Work out the finished part from the listing and answer in its coordinate system (mm). A direction names the side the tool comes from. Coordinates: 2 decimals unless noted, no trailing zeros. Write each loop counter-clockwise with the first axis right and the second up, starting at its lowest first coordinate (ties: lowest second). Pieces come first, ordered by that corner, then holes. Notation, with made-up numbers: (64.5, 23) - (92.5, 23) arc R14 ccw to (92.5, 48) - close; hole circle Ø3 at (7.5, 76.5). An arc over 180 degrees is marked (long way). Answer as a JSON object with one key per item and string values. Group by question number.
from build123d import *

# Parameters (mm, degrees)
SKETCH1_R           = 1.5999999999999992
SKETCH1_R_2         = 1.6
BOSS_EXTRUDE1_DEPTH = 1.5
BOSS_EXTRUDE2_DEPTH = 20
FILLET1_R           = 5
SKETCH2_R           = 1.6500000000000017
SKETCH2_W           = 42.900000000000006
SKETCH2_H           = 21.999999999999993
CUT_EXTRUDE1_DEPTH  = 191.86971996626394
FILLET2_R           = 2


with BuildPart() as part:
    # Sketch1 → Boss-Extrude1 (new, symmetric)
    with BuildSketch(Plane(origin=(0, 0, 0), x_dir=(1, 0, 0), z_dir=(0, 1, 0))):
        Polygon((-15, -39), (-15, 39), (-14.999999999999993, 64), (5.358274547724965, 122.5), (119.64234676884817, 122.50000000000003), (145.00000000000003, 86.28551808227317), (145.00000000000003, -86.28551808227317), (119.64234676884817, -122.50000000000003), (5.358274547725049, -122.49999999999999), (-14.999999999999993, -64), align=None)
        with Locations(Location((0, 31, 0), (0, 0, 270))):
            Circle(SKETCH1_R, mode=Mode.SUBTRACT)
        with Locations(Location((0, -31, 0), (0, 0, 90))):
            Circle(SKETCH1_R_2, mode=Mode.SUBTRACT)
        Polygon((25.197972880423116, 27.499999999999996), (128, 27.499999999999996), (128, 80.92543867133034), (110.7927069094685, 105.50000000000004), (17.442194764625423, 105.50000000000001), (3.0000000000000027, 64), (3.0000000000000027, 39), align=None, mode=Mode.SUBTRACT)
        Polygon((25.197972880423116, -27.499999999999996), (128, -27.499999999999996), (128, -80.92543867133034), (110.7927069094685, -105.50000000000004), (17.442194764625537, -105.49999999999999), (3.0000000000000027, -64), (3.0000000000000027, -39), align=None, mode=Mode.SUBTRACT)
    extrude(amount=BOSS_EXTRUDE1_DEPTH, both=True)

    # Sketch3 → Boss-Extrude2 (add)
    with BuildSketch(Plane(origin=(0, 1.5, 0), x_dir=(1, 0, 0), z_dir=(0, 1, 0))):
        Polygon((120.00000000000004, -2.999999999999993), (120.00000000000004, 3.0000000000000075), (138, 3.0000000000000075), (138, 84.07842656012029), (115.99837741498601, 115.49999999999999), (10.334006401742785, 115.49999999999997), (-4.464169294218266, 72.97708008435012), (-11.07528040532939, 75.27777777777771), (5.358274547724965, 122.5), (119.64234676884817, 122.50000000000003), (145.00000000000003, 86.28551808227317), (145.00000000000003, -86.28551808227317), (119.64234676884817, -122.50000000000003), (5.358274547724965, -122.5), (-11.075280405329384, -75.27777777777771), (-4.464169294218257, -72.97708008435012), (10.334006401742798, -115.49999999999997), (115.99837741498602, -115.49999999999996), (138, -84.07842656012026), (138, -2.999999999999991), align=None)
    extrude(amount=BOSS_EXTRUDE2_DEPTH)

    # Fillet1
    fillet1_edges = [part.edges().sort_by_distance(p)[0] for p in [
        (115.99837741498602, 11.5, 115.49999999999996),
        (10.334006401742798, 11.5, 115.49999999999997),
        (-11.075280405329384, 11.5, 75.27777777777771),
        (-11.07528040532939, 11.5, -75.27777777777771),
        (10.334006401742785, 11.5, -115.49999999999997),
        (115.99837741498601, 11.5, -115.49999999999999),
        (138, 11.5, -84.07842656012029),
        (5.358274547724965, 10, -122.5),
        (119.64234676884817, 10, -122.50000000000003),
        (145.00000000000003, 10, -86.28551808227317),
        (145.00000000000003, 10, 86.28551808227317),
        (119.64234676884817, 10, 122.50000000000003),
        (5.358274547725006, 10, 122.5),
        (128, 0, -80.92543867133034),
        (110.7927069094685, 0, -105.50000000000004),
        (17.442194764625423, 0, -105.50000000000001),
        (138, 11.5, -3.0000000000000075),
        (138, 11.5, 2.999999999999991),
        (138, 11.5, 84.07842656012026),
    ]]
    fillet(fillet1_edges, radius=FILLET1_R)

    # Sketch2 → Cut-Extrude1 (cut, through all)
    with BuildSketch(Plane(origin=(0, 1.5, 0), x_dir=(1, 0, 0), z_dir=(0, 1, 0))):
        with Locations(Location((56.999999999999964, 18.99999999999999, 0), (0, 0, 270))):
            Circle(SKETCH2_R)
        with Locations(Location((84.99999999999997, 18.999999999999993, 0), (0, 0, 270))):
            Circle(SKETCH2_R)
        with Locations(Location((101.99999999999999, 16.999999999999996, 0), (0, 0, 270))):
            Circle(SKETCH2_R)
        with Locations(Location((101.99999999999999, -16.999999999999996, 0), (0, 0, 90))):
            Circle(SKETCH2_R)
        with Locations(Location((84.99999999999997, -18.999999999999993, 0), (0, 0, 90))):
            Circle(SKETCH2_R)
        with Locations(Location((56.999999999999964, -18.99999999999999, 0), (0, 0, 90))):
            Circle(SKETCH2_R)
        with Locations((81.24999999999999, 3.819e-14)):
            Rectangle(SKETCH2_W, SKETCH2_H)
    extrude(amount=-CUT_EXTRUDE1_DEPTH, mode=Mode.SUBTRACT)

    # Fillet2
    fillet2_edges = [part.edges().sort_by_distance(p)[0] for p in [
        (59.79999999999998, 0, -11.000000000000036),
        (102.69999999999999, 0, -11.000000000000036),
        (102.69999999999999, 0, 10.99999999999996),
        (59.79999999999998, 0, 10.99999999999996),
    ]]
    fillet(fillet2_edges, radius=FILLET2_R)


solid = part.part
Q1. Section C-C on z = -36 is taken. Determine the outline of the cut face in (x, y), plus the area to 3 significant figures.
Q2. Section D-D on z = -98.5 is taken. Determine the outline of the cut face in (x, y).
Q3. For a pull along Z with two mould halves and no side action, classify faces 1 (the face through (127.16, 11.36, 99.56)), 2 (the face through (132.455, 9.839, -104.202)), 3 (the face through (13.944, 0.021, -33.33)), 4 (the face through (5.98, 10.16, 121.55)) as +Z half, -Z half, draft (parallel to the pull), parting line (faces both ways), or undercut.
Q4. Section B-B on x = 47 is taken. Determine the outline of the cut face in (y, z).
Q5. Flat-ended cylindrical pins translate along their axes: pin 1 Ø2 at (x, z) = (102, -17) entering from -Y; pin 2 Ø4 at (x, z) = (0, -31) entering from +Y; pin 3 Ø6 at (y, z) = (12, 17.5) entering from -X; pin 4 Ø3 at (y, z) = (12, -0.5) entering from -X. Find the tip coordinate at first contact, or state that the pin passes through.
Q6. Consider L1, parallel to X at y = 0.7, z = -19; L2, parallel to Z at x = 96, y = 12.25; L3, parallel to Z at x = 57, y = -0.25. Determine where each line is inside the solid, lowest interval first. Write a range as from..to.
Q7. Section A-A on z = 59.5 is taken. Determine the outline of the cut face in (x, y).
Q8. A tool of negligible diameter and unlimited length cuts with its end or side. For faces 5 (the face through (-9.187, 11.64, 76.13)), 6 (the face through (63, 11, 115.5)), 7 (the face through (10.32, 0.02, 85.04)), from which of +Z, -Z, +X, -X, +Y, -Y can it reach the whole face along a straight path? Write none if from no direction.
Numbers:
{
 "1": {"outline": "(-15, -1.5) - (8.79, -1.5) - (8.79, 1.5) - (-15, 1.5) - close; (128, -1.5) - (145, -1.5) - (145, 21.5) - (138, 21.5) - (138, 1.5) - (128, 1.5) - close", "area": "262 mm²"},
 "2": {"outline": "(-2.99, -1.5) - (15.01, -1.5) - (15.01, 1.5) - (4.42, 1.5) - (4.42, 21.5) - (-2.99, 21.5) - close; (115.69, -1.5) - (136.45, -1.5) - (136.45, 21.5) - (127.9, 21.5) - (127.9, 1.5) - (115.69, 1.5) - close"},
 "3": {"face 1": "undercut", "face 2": "-Z half", "face 3": "undercut", "face 4": "+Z half"},
 "4": {"outline": "(-1.5, -122.5) - (21.5, -122.5) - (21.5, -115.5) - (1.5, -115.5) - (1.5, -105.5) - (-1.5, -105.5) - close; (-1.5, -27.5) - (1.5, -27.5) - (1.5, 27.5) - (-1.5, 27.5) - close; (-1.5, 105.5) - (1.5, 105.5) - (1.5, 115.5) - (21.5, 115.5) - (21.5, 122.5) - (-1.5, 122.5) - close"},
 "5": {"pin 1": "passes through", "pin 2": "stops at y = 1.5", "pin 3": "stops at x = 138", "pin 4": "stops at x = 120"},
 "6": {"L1": "x = -15..55.35, 58.65..83.35, 86.65..145", "L2": "z = -122.5..-115.5, 115.5..122.5", "L3": "z = -122.5..-105.5, -27.5..-20.65, -17.35..17.35, 20.65..27.5, 105.5..122.5"},
 "7": {"outline": "(-15, -1.5) - (3, -1.5) - (3, 1.5) - (-15, 1.5) - close; (128, -1.5) - (145, -1.5) - (145, 21.5) - (138, 21.5) - (138, 1.5) - (128, 1.5) - close"},
 "8": {"face 5": "-X, +Y", "face 6": "+Y", "face 7": "+Y, -Y"}
}
